Model file for the job. Use its own axes, mm. A direction names the side the tool comes from. Round coordinates to 2 decimals unless told otherwise and drop trailing zeros. Order: outer loops, then holes, each group sorted by start corner. A loop starts at its lowest first (then second) coordinate and runs counter-clockwise, first axis right, second up. Notation, with made-up numbers: (84.5, 49.5) - (116.5, 49.5) arc R18 ccw to (116.5, 54.5) - close; hole circle Ø8 at (-12, 83). An arc over 180 degrees is marked (long way). Use one line per item in the form item = value.
from build123d import *

# Parameters (mm, degrees)
F0_W     = 76.2
F0_H     = 50.8
F0_R     = 12.7
F1_DEPTH = 29.972
F2_W     = 6.35
F2_H     = 50.8
F3_DEPTH = 2.54
F5_R     = 10.6886157163
F6_DEPTH = 25.4
F7_DEPTH = 50.801


with BuildPart() as f1:
    # F0 (on Top) → F1 (new body)
    with BuildSketch(Plane.XY):
        with Locations((3.3417083323, 0.1945786622)):
            Rectangle(F0_W, F0_H)
        with Locations((2.0050231833, 0)):
            Circle(F0_R, mode=Mode.SUBTRACT)
    extrude(amount=F1_DEPTH)

    # F2 (on face) → F3 (cut)
    with BuildSketch(Plane.XY.offset(29.972)):
        with Locations((-29.0432916677, 0.1945786622)):
            Rectangle(F2_W, F2_H)
        with BuildLine():
            Line((6.35, 25.5945786622), (-6.35, 25.5945786622))
            Line((-6.35, 25.5945786622), (-6.35, 9.5647053068))
            ThreePointArc((-6.35, 9.5647053068), (-0.3237214829, 12.484668529), (6.35, 11.9336153978))
            Line((6.35, 11.9336153978), (6.35, 25.5945786622))
        make_face()
        with BuildLine():
            Line((-6.35, -9.5647053068), (-6.35, -25.2054213378))
            Line((-6.35, -25.2054213378), (6.35, -25.2054213378))
            Line((6.35, -25.2054213378), (6.35, -11.9336153978))
            ThreePointArc((6.35, -11.9336153978), (-0.3237214829, -12.484668529), (-6.35, -9.5647053068))
        make_face()
    extrude(amount=-F3_DEPTH, mode=Mode.SUBTRACT)

    # F5 (on face) → F6 (join)
    with BuildSketch(Plane.YZ.offset(41.4417083323)):
        with Locations((0.1945786622, 14.986)):
            Circle(F5_R)
    extrude(amount=F6_DEPTH)

    # F4 (on face) → F7 (cut, through all)
    with BuildSketch(Plane.XZ.offset(25.2054213378)):
        Polygon((36.5958541662, 29.972), (23.8958541662, 29.972), (20.9629147987, 24.892), (39.5287935336, 24.892), align=None)
    extrude(amount=-F7_DEPTH, mode=Mode.SUBTRACT)


solid = f1.part
(1) Tool access for faces 1 (the face through (-29, 1, 27.432)), 2 (the face through (53.96, 5.94, 24)), 3 (the face through (38.08, -0.16, 27.4)): list every direction of +Z, -Z, +X, -X, +Y, -Y with a clear straight run to the whole face (end or side of a thin tool).
Report:
face_1 = +Z, +Y, -Y
face_2 = +X
face_3 = +Y, -Y
(2) Slice it at C-C on z = 20. Give the cut face in (x, y).
Report:
outline = (-34.76, -25.21) - (41.44, -25.21) - (41.44, -9.25) - (66.84, -9.25) - (66.84, 9.63) - (41.44, 9.63) - (41.44, 25.59) - (-34.76, 25.59) - close; hole circle Ø25.4 at (2.01, 0)
(3) Probe probe 1 along Z at (x, y) = (-5, -20.5); probe 2 along X at (y, z) = (-19, 2.5); probe 3 along Y at (x, z) = (-2, 15). List the from-to ranges inside material, lowest first. Write a range as [from, to].
Report:
probe_1 = [0, 27.43]
probe_2 = [-34.76, 41.44]
probe_3 = [-25.21, -12.05], [12.05, 25.59]
(4) Pull direction Z, two halves, no side cores. Call faces 4 (the face through (-6, 12, 0)), 5 (the face through (22.45, -0.16, 27.47)), 6 (the face through (0, 19, 27.432)): released by +Z, released by -Z, zero draft, split by the parting line, or undercut.
Report:
face_4 = released by -Z
face_5 = undercut
face_6 = released by +Z
(5) Pin check, flat tips, straight feed: pin 1 (1 mm diameter, centred on x = 16, y = 3.5, fed in from -Z); pin 2 (2 mm diameter, centred on y = -5, z = 29.5, fed in from +X); pin 3 (1.5 mm diameter, centred on x = 54, z = 21, fed in from +Y); pin 4 (6.5 mm diameter, centred on x = 0.5, y = -14.5, fed in from +Z). Stop position of each tip, or through.
Report:
pin_1 = 0
pin_2 = 41.44
pin_3 = 9.5
pin_4 = 27.43
(6) Slice it at A-A on y = 16.5. Give the cut face in (x, z).
Report:
outline = (-34.76, 0) - (41.44, 0) - (41.44, 29.97) - (36.6, 29.97) - (39.53, 24.89) - (20.96, 24.89) - (23.9, 29.97) - (6.35, 29.97) - (6.35, 27.43) - (-6.35, 27.43) - (-6.35, 29.97) - (-25.87, 29.97) - (-25.87, 27.43) - (-32.22, 27.43) - (-32.22, 29.97) - (-34.76, 29.97) - close
(7) Slice it at D-D on y = 0. Give the cut face in (x, z).
Report:
outline = (-34.76, 0) - (-10.69, 0) - (-10.69, 29.97) - (-25.87, 29.97) - (-25.87, 27.43) - (-32.22, 27.43) - (-32.22, 29.97) - (-34.76, 29.97) - close; (14.71, 0) - (41.44, 0) - (41.44, 4.3) - (66.84, 4.3) - (66.84, 25.67) - (41.44, 25.67) - (41.44, 29.97) - (36.6, 29.97) - (39.53, 24.89) - (20.96, 24.89) - (23.9, 29.97) - (14.71, 29.97) - close
(8) Slice it at B-B on x = -9. Give the cut face in (y, z).
Report:
outline = (-25.21, 0) - (-6.34, 0) - (-6.34, 29.97) - (-25.21, 29.97) - close; (6.34, 0) - (25.59, 0) - (25.59, 29.97) - (6.34, 29.97) - close
